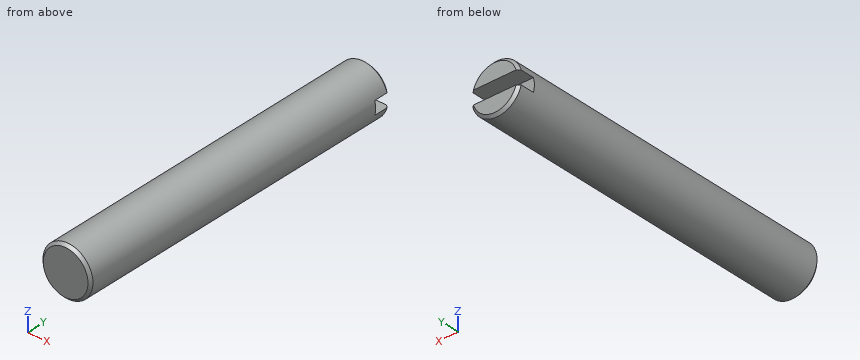
```python
from build123d import *

# Parameters (mm, degrees)
SKETCH1_R           = 1.875
BOSS_EXTRUDE1_DEPTH = 25.63
CHAMFER1_SIZE       = 0.2
CHAMFER2_SIZE       = 0.2
SKETCH2_W           = 3.856306074
SKETCH2_H           = 1
CUT_EXTRUDE1_DEPTH  = 1.25


with BuildPart() as part:
    # Sketch1 → Boss-Extrude1 (new body)
    with BuildSketch(Plane(origin=(0, 0, 0), x_dir=(1, 0, 0), z_dir=(0, 1, 0))):
        Circle(SKETCH1_R)
    extrude(amount=BOSS_EXTRUDE1_DEPTH)

    # Chamfer1
    chamfer1_edges = [part.edges().sort_by_distance(p)[0] for p in [
        (-1.875, 25.63, 0),
    ]]
    chamfer(chamfer1_edges, length=CHAMFER1_SIZE)

    # Chamfer2
    chamfer2_edges = [part.edges().sort_by_distance(p)[0] for p in [
        (-1.875, 0, 0),
    ]]
    chamfer(chamfer2_edges, length=CHAMFER2_SIZE)

    # Sketch2 → Cut-Extrude1 (cut)
    with BuildSketch(Plane(origin=(0, 25.63, 0), x_dir=(1, 0, 0), z_dir=(0, 1, 0))):
        Rectangle(SKETCH2_W, SKETCH2_H)
    extrude(amount=-CUT_EXTRUDE1_DEPTH, mode=Mode.SUBTRACT)


solid = part.part
```
For this review, take the finished solid that the model builds, in its own axes (mm). Round coordinates to 2 decimals unless told otherwise and drop trailing zeros. Write each loop counter-clockwise with the first axis right and the second up, starting at its lowest first coordinate (ties: lowest second). Pieces come first, ordered by that corner, then holes. Notation, with made-up numbers: (-30, -28.75) -> (2, -28.75) arc R14 ccw to (2, -22.75) -> close; hole circle Ø11 at (-30.75, -9). An arc over 180 degrees is marked (long way). Use one line per item in the form item = value.
1) Take a section at B-B, the plane y = 18. Write out the cut boundary in (x, z) (3 decimals), and give its area (3 significant figures).
Found:
outline = circle Ø3.75 at (0, 0)
area = 11.0 mm2
2) Clearance check with flat-ended pins moving along their axes: pin 1 (0.6 mm diameter, centred on x = -0.5, y = 25, fed in from +Z); pin 2 (0.5 mm diameter, centred on x = 0.5, z = 0, fed in from +Y); pin 3 (0.6 mm diameter, centred on x = -0.5, y = 25, fed in from -Z). State where each tip first meets the part, or that it passes through.
Found:
pin_1 = 1.86
pin_2 = 24.38
pin_3 = -1.86
3) Take a section at A-A, the plane z = 0. Write out the cut boundary in (x, y) (3 decimals), and give its area (3 significant figures).
Found:
outline = (-1.875, 0.2) -> (-1.675, 0) -> (1.675, 0) -> (1.875, 0.2) -> (1.875, 24.38) -> (-1.875, 24.38) -> close
area = 91.4 mm2
4) To check wall thickness, follow L1, parallel to Z at x = -0.1, y = 21; L2, parallel to Y at x = -0.6, z = 0.3; L3, parallel to Z at x = -0.5, y = 8.25. State the ranges of each line that lie inside material, in increasing order. Write a range as from..to.
Found:
L1 = -1.87..1.87
L2 = 0..24.38
L3 = -1.81..1.81
